from build123d import *

# Parameters (mm, degrees)
F0_R     = 10.5
F1_DEPTH = 4
F2_R     = 8
F3_DEPTH = 39
F4_W     = 7
F4_H     = 5
F6_R     = 1.5
F7_DEPTH = 47.7


with BuildPart() as f1:
    # F0 (on Top) → F1 (new body)
    with BuildSketch(Plane.XY):
        Circle(F0_R)
    extrude(amount=F1_DEPTH)

    # F2 (on Top) → F3 (join)
    with BuildSketch(Plane.XY):
        Circle(F2_R)
    extrude(amount=F3_DEPTH)

    # F4 (on Right) → F5 (revolve)
    with BuildSketch(Plane.YZ):
        with Locations((3.5, 41.5)):
            Rectangle(F4_W, F4_H)
    revolve(axis=Axis((0, 0, 41.5), (0, 0, -1)))

    # F6 (on face) → F7 (cut)
    with BuildSketch(Plane.XY.offset(44)):
        Circle(F6_R)
    extrude(amount=-F7_DEPTH, mode=Mode.SUBTRACT)


solid = f1.part
Work out the finished part from the listing and answer in its coordinate system (mm). A direction names the side the tool comes from. Round coordinates to 2 decimals unless told otherwise and drop trailing zeros. Write each loop counter-clockwise with the first axis right and the second up, starting at its lowest first coordinate (ties: lowest second). Pieces come first, ordered by that corner, then holes.
1) A cutting plane is placed at D-D (x = 4). Give the vertices of the cut face in (y, z), plus the area to 3 significant figures.
2) Given pin 1 Ø1.5 at (y, z) = (0, 30) entering from -X; pin 2 Ø1.5 at (x, z) = (2, 24.5) entering from +Y; pin 3 Ø1 at (y, z) = (-7.5, 29) entering from -X, each flat-ended and moving along its own axis, determine where each tip first touches the part or whether it passes through.
3) The mould has two halves that part along X. Classify faces 1 (the cylindrical face through (-2.681, 6.466, 41.535)), 2 (the cylindrical face through (-1.5, 0.07, 22.31)), 3 (the flat face through (4, -6, 39)): pulls with the +X half, pulls with the -X half, needs draft (parallel to the pull), parting line crosses it, or undercut.
4) A cutting plane is placed at C-C (y = 4.25). Give the vertices of the cut face in (x, z).
5) Straight lines are drawn through the part: line 1 (Y direction, x = 0, z = 22); line 2 (Y direction, x = -1, z = 14); line 3 (Z direction, x = -5, y = -8.75). For each, find the intervals that lie inside material, in ascending order.
6) A cutting plane is placed at A-A (y = 0). Give the vertices of the cut face in (x, z).
7) A tool of negligible diameter and unlimited length cuts with its end or side. For faces 4 (the cylindrical face through (10, 3.2, 2)), 5 (the flat face through (-2, -8, 4)), from which of +Z, -Z, +X, -X, +Y, -Y can it reach the whole face along a straight path? Write none if from no direction.
Completed:
1. outline: (-9.71, 0) - (9.71, 0) - (9.71, 4) - (6.93, 4) - (6.93, 39) - (5.74, 39) - (5.74, 44) - (-5.74, 44) - (-5.74, 39) - (-6.93, 39) - (-6.93, 4) - (-9.71, 4) - close
1. area: 620 mm2
2. pin 1: stops at x = -8
2. pin 2: stops at y = 7.9
2. pin 3: stops at x = -3.87
3. face 1: parting line crosses it
3. face 2: undercut
3. face 3: needs draft
4. outline: (-9.6, 0) - (9.6, 0) - (9.6, 4) - (6.78, 4) - (6.78, 39) - (5.56, 39) - (5.56, 44) - (-5.56, 44) - (-5.56, 39) - (-6.78, 39) - (-6.78, 4) - (-9.6, 4) - close
5. line 1: y = -8 to -1.5, 1.5 to 8
5. line 2: y = -7.94 to -1.12, 1.12 to 7.94
5. line 3: z = 0 to 4
6. outline: (-10.5, 0) - (-1.5, 0) - (-1.5, 44) - (-7, 44) - (-7, 39) - (-8, 39) - (-8, 4) - (-10.5, 4) - close; (1.5, 0) - (10.5, 0) - (10.5, 4) - (8, 4) - (8, 39) - (7, 39) - (7, 44) - (1.5, 44) - close
7. face 4: +Z, -Z
7. face 5: +Z
